Part model, mm, in its own coordinate system. A direction names the side the tool comes from. Give positions to 0.01 mm unless a question says otherwise; leave off trailing zeros. Order: outer loops, then holes, each group sorted by start corner. A loop starts at its lowest first (then second) coordinate and runs counter-clockwise, first axis right, second up. Notation, with made-up numbers: (75, 68.25) -> (83, 68.25) arc R30 ccw to (83, 101.25) -> close; hole circle Ø2 at (19, -6.75). An arc over 180 degrees is marked (long way). Write item = value, one per line. Start each with the question number.
(1) Flat gauge pin, fed straight in: pin 1 (2.5 mm diameter, centred on x = 0, y = 112, fed in from +Z). Where does the tip first touch, or does it go through?
(2) Two-plate mould, pull along X, no slides. Class faces 1 (the cylindrical face through (-0.481, 21.474, 6.993)), 2 (the flat face through (0, 59, -7.5)), 3 (the flat face through (7.5, 59, 0)): pulls with the +X half, pulls with the -X half, needs draft (parallel to the pull), parting line crosses it, or undercut.
(3) Saw through at D-D, the plane y = 97. List the corners of the cut face in (x, z).
(4) Saw through at B-B, the plane z = -2.25. List the corners of the cut face in (x, y), then the cut area to 3 significant figures.
(5) Which spindle directions (+Z, -Z, +X, -X, +Y, -Y) get a long thin tool onto all of the face, cutting with end or side? Do faces 4 (the flat face through (0, 59, 6.5)), 5 (the cylindrical face through (-0.481, 21.474, -7.007)). Say none if no direction does.
(6) Probe line 1 along Y through (x, z) = (0, -7.2); line 2 along X through (y, z) = (97, 7.2); line 3 along Z through (x, y) = (3.5, 87). List the from-to ranges inside material, lowest first. Write a range as from..to.
(7) Saw through at A-A, the plane x = -4.5. List the corners of the cut face in (y, z).
(8) Saw through at C-C, the plane y = 74. List the corners of the cut face in (x, z), then the cut area to 3 significant figures.
Autodesk Inventor part; units mm, degrees
ref_plane "YZ Plane" through (0, 0, 0) normal (1, 0, 0) x (0, 1, 0)
ref_plane "XZ Plane" through (0, 0, 0) normal (0, 1, 0) x (-1, 0, 0)
ref_plane "XY Plane" through (0, 0, 0) normal (0, 0, 1) x (1, 0, 0)
sketch "スケッチ1" plane through (0, 0, 0) normal (0, 1, 0) x (-1, 0, 0)
  line L0 (7.5, -7.5) -> (-7.5, -7.5)
  line L1 (-7.5, -7.5) -> (-7.5, 7.5)
  line L2 (-7.5, 7.5) -> (7.5, 7.5)
  line L3 (7.5, 7.5) -> (7.5, -7.5)
  line L4 (7.5, -7.5) -> (-7.5, 7.5) construction
  line L5 (-7.5, -7.5) -> (7.5, 7.5) construction
  point P0 (0, 0)
  dimension "d0" = 15
  dimension "d1" = 15
extrude "押し出し1" add sketch "スケッチ1" along normal blind 120
shell "シェル1" thickness 1 removed faces 2 at (-2.5, 0, -2.5) at (-2.5, 120, -2.5)
sketch "スケッチ2" plane through (-7.5, 0, 7.5) normal (0, 0, 1) x (1, 0, 0)
  line L0 (15, 0) -> (0, 0)
  line L1 (0, 120) -> (15, 120)
  point P0 (7.5, 0)
  point P1 (7.5, 8)
  point P2 (7.5, 23)
  point P3 (7.5, 0)
  point P4 (7.5, 112)
  point P5 (7.5, 97)
  point P6 (7.5, 120)
  dimension "d5" = 8
  dimension "d6" = 15
  dimension "d14" = 8
  dimension "d15" = 15
hole "穴1" at (0, 8, 7.5) at (0, 23, 7.5) at (0, 112, 7.5) at (0, 97, 7.5) direction (0, 0, -1) diameter 3.2 end through all
properties part number "PitchSquarePipe" material "アルミニウム 5005-H12"
Results list:
q1.pin_1 = through
q2.face_1 = undercut
q2.face_2 = needs draft
q2.face_3 = pulls with the +X half
q3.outline = (-7.5, -7.5) -> (-1.6, -7.5) -> (-1.6, -6.5) -> (-6.5, -6.5) -> (-6.5, 6.5) -> (-1.6, 6.5) -> (-1.6, 7.5) -> (-7.5, 7.5) -> close; (1.6, -7.5) -> (7.5, -7.5) -> (7.5, 7.5) -> (1.6, 7.5) -> (1.6, 6.5) -> (6.5, 6.5) -> (6.5, -6.5) -> (1.6, -6.5) -> close
q4.outline = (-7.5, 0) -> (-6.5, 0) -> (-6.5, 120) -> (-7.5, 120) -> close; (6.5, 0) -> (7.5, 0) -> (7.5, 120) -> (6.5, 120) -> close
q4.area = 240 mm^2
q5.face_4 = +Y, -Y
q5.face_5 = +Z, -Z
q6.line_1 = 0..6.4, 9.6..21.4, 24.6..95.4, 98.6..110.4, 113.6..120
q6.line_2 = -7.5..-1.6, 1.6..7.5
q6.line_3 = -7.5..-6.5, 6.5..7.5
q7.outline = (0, -7.5) -> (120, -7.5) -> (120, -6.5) -> (0, -6.5) -> close; (0, 6.5) -> (120, 6.5) -> (120, 7.5) -> (0, 7.5) -> close
q8.outline = (-7.5, -7.5) -> (7.5, -7.5) -> (7.5, 7.5) -> (-7.5, 7.5) -> close; hole (-6.5, -6.5) -> (6.5, -6.5) -> (6.5, 6.5) -> (-6.5, 6.5) -> close
q8.area = 56.0 mm^2
